from build123d import *

# Parameters (mm, degrees)
SKETCH_4_W          = 3
SKETCH_4_H          = 3
EXTRUDE_1_DEPTH     = 22
SKETCH_4_5_R        = 0.7
CUT_EXTRUDE_1_DEPTH = 3
CUT_EXTRUDE_START   = 19
SKETCH_4_6_R        = 0.7
CUT_EXTRUDE_2_DEPTH = 3


with BuildPart() as part:
    # 草图4 → 凸台-拉伸1 (new body)
    with BuildSketch(Plane(origin=(0, 0, 0), x_dir=(1, 0, 0), z_dir=(0, 1, 0))):
        Rectangle(SKETCH_4_W, SKETCH_4_H)
    extrude(amount=EXTRUDE_1_DEPTH)

    # 草图4<5> → 切除-拉伸1 (cut)
    with BuildSketch(Plane(origin=(0, 0, 0), x_dir=(1, 0, 0), z_dir=(0, 1, 0))):
        with Locations(Location((0, 0, 0), (0, 0, 270))):
            Circle(SKETCH_4_5_R)
    extrude(amount=CUT_EXTRUDE_1_DEPTH, mode=Mode.SUBTRACT)

    # 草图4<6> → 切除-拉伸2 (cut)
    with BuildSketch(Plane(origin=(0, 0, 0), x_dir=(1, 0, 0), z_dir=(0, 1, 0)).offset(CUT_EXTRUDE_START)):
        with Locations(Location((0, 0, 0), (0, 0, 270))):
            Circle(SKETCH_4_6_R)
    extrude(amount=CUT_EXTRUDE_2_DEPTH, mode=Mode.SUBTRACT)


solid = part.part
The listing builds one solid part. Answer for the finished solid, in the listing's coordinates (mm). A direction names the side the tool comes from. Round coordinates to 2 decimals unless told otherwise and drop trailing zeros. Write each loop counter-clockwise with the first axis right and the second up, starting at its lowest first coordinate (ties: lowest second). Pieces come first, ordered by that corner, then holes. Notation, with made-up numbers: (75.25, -19.75) - (120.25, -19.75) arc R15 ccw to (120.25, -15.75) - close; hole circle Ø10 at (3, -20). An arc over 180 degrees is marked (long way). Use one line per item in the form item = value. Start each with the question number.
Item 1: A cutting plane is placed at A-A (x = 0). Write down the section's boundary in (y, z).
Item 2: A tool of negligible diameter and unlimited length cuts with its end or side. For faces 4 (the cylindrical face through (0, 20.5, -0.7)), 5 (the flat face through (0, 3, 0)), 6 (the flat face through (1, 22, 0)), from which of +Z, -Z, +X, -X, +Y, -Y can it reach the whole face along a straight path? Write none if from no direction.
Item 3: Find the intervals of material crossed by line 1 (Z direction, x = -0.45, y = 2.5); line 2 (Z direction, x = -0.55, y = 2.5); line 3 (X direction, y = 1.95, z = 0), in increasing order. Write a range as [from, to].
Item 4: A flat-ended cylindrical pin translates along its axis: pin 1 Ø1.1 at (x, z) = (0, 0) entering from +Y. Find the tip coordinate at first contact, or state that the pin passes through.
Item 5: A cutting plane is placed at B-B (z = 0). Write down the section's boundary in (x, y).
Item 6: Determine the mould class of faces 1 (the cylindrical face through (0, 1.5, -0.7)), 2 (the flat face through (1.5, 11, 0)), 3 (the flat face through (0, 11, 1.5)) for opening direction Z: +Z half, -Z half, draft (parallel to the pull), parting line (faces both ways), or undercut.
The answers:
q1.outline = (0, -1.5) - (22, -1.5) - (22, -0.7) - (19, -0.7) - (19, 0.7) - (22, 0.7) - (22, 1.5) - (0, 1.5) - (0, 0.7) - (3, 0.7) - (3, -0.7) - (0, -0.7) - close
q2.face_4 = +Y
q2.face_5 = -Y
q2.face_6 = +Z, -Z, +X, -X, +Y
q3.line_1 = [-1.5, -0.54], [0.54, 1.5]
q3.line_2 = [-1.5, -0.43], [0.43, 1.5]
q3.line_3 = [-1.5, -0.7], [0.7, 1.5]
q4.pin_1 = 19
q5.outline = (-1.5, 0) - (-0.7, 0) - (-0.7, 3) - (0.7, 3) - (0.7, 0) - (1.5, 0) - (1.5, 22) - (0.7, 22) - (0.7, 19) - (-0.7, 19) - (-0.7, 22) - (-1.5, 22) - close
q6.face_1 = undercut
q6.face_2 = draft
q6.face_3 = +Z half
